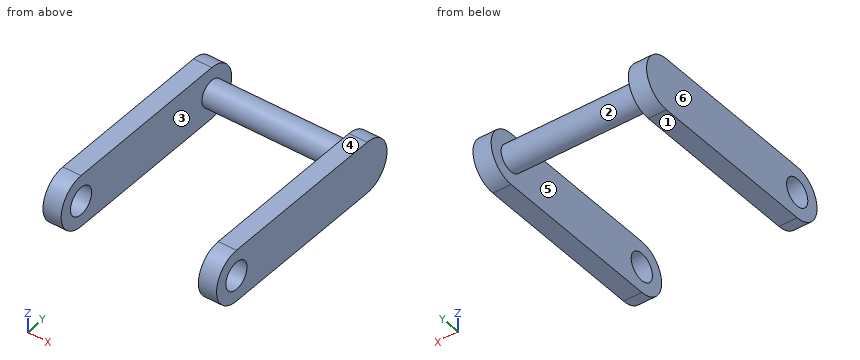
```python
from build123d import *

# Parameters (mm, degrees)
PAD139_DEPTH            = 2
SKETCH244_R             = 1.5
PAD140_DEPTH            = 16
PAD141_DEPTH            = 2
SKETCH246_R             = 1.5
PAD142_DEPTH            = 0.5
SKETCH247_R             = 1.5
PAD143_DEPTH            = 0.5
PAD143_FACE5_R          = 1.5
PAD212_DEPTH            = 0.1
PAD212_FACE4_R          = 1.5
PAD213_DEPTH            = 0.1
SKETCH353_R             = 1.6
POCKET170_DEPTH         = 22
BODY020_ROLL_ANGLE      = 90
BODY020_PLACEMENT_ANGLE = 90


with BuildPart() as part:
    # Sketch243 → Pad139 (new body)
    with BuildSketch(Plane.XY):
        with BuildLine():
            ThreePointArc((0, 3), (-3, 0), (0, -3))
            Line((0, -3), (19.75, -3))
            ThreePointArc((19.75, -3), (22.75, 0), (19.75, 3))
            Line((0, 3), (19.75, 3))
        make_face()
    extrude(amount=PAD139_DEPTH)

    # Sketch244 (on Face6 of Pad139) → Pad140 (join)
    with BuildSketch(Plane.XY.offset(2)):
        Circle(SKETCH244_R)
        with Locations((19.75, 0)):
            Circle(SKETCH244_R)
    extrude(amount=PAD140_DEPTH)

    # Sketch245 (on Face9 of Pad140) → Pad141 (join)
    with BuildSketch(Plane.XY.offset(18)):
        with BuildLine():
            ThreePointArc((0, 3), (-3, 0), (0, -3))
            Line((0, -3), (19.75, -3))
            ThreePointArc((19.75, -3), (22.75, 0), (19.75, 3))
            Line((0, 3), (19.75, 3))
        make_face()
    extrude(amount=PAD141_DEPTH)

    # Sketch246 (on Face14 of Pad141) → Pad142 (join)
    with BuildSketch(Plane.XY.offset(20)):
        Circle(SKETCH246_R)
    extrude(amount=PAD142_DEPTH)

    # Sketch247 (on Face4 of Pad142) → Pad143 (join)
    with BuildSketch(Plane(origin=(0, 0, 0), x_dir=(1, 0, 0), z_dir=(0, 0, -1))):
        Circle(SKETCH247_R)
    extrude(amount=PAD143_DEPTH)

    # Pad143 Face5 → Pad212 (add)
    with BuildSketch(Plane(origin=(9.875, 0, 2), x_dir=(0, 1, 0), z_dir=(0, 0, 1))):
        with BuildLine():
            ThreePointArc((3, 9.875), (0, 12.875), (-3, 9.875))
            Line((-3, 9.875), (-3, -9.875))
            ThreePointArc((-3, -9.875), (0, -12.875), (3, -9.875))
            Line((3, -9.875), (3, 9.875))
        make_face()
        with Locations((0, 9.875)):
            Circle(PAD143_FACE5_R, mode=Mode.SUBTRACT)
        with Locations((0, -9.875)):
            Circle(PAD143_FACE5_R, mode=Mode.SUBTRACT)
    extrude(amount=PAD212_DEPTH)

    # Pad212 Face4 → Pad213 (add)
    with BuildSketch(Plane(origin=(9.875, 0, 18), x_dir=(0, -1, 0), z_dir=(0, 0, -1))):
        with BuildLine():
            ThreePointArc((3, 9.875), (0, 12.875), (-3, 9.875))
            Line((-3, 9.875), (-3, -9.875))
            ThreePointArc((-3, -9.875), (0, -12.875), (3, -9.875))
            Line((3, -9.875), (3, 9.875))
        make_face()
        with Locations((0, 9.875)):
            Circle(PAD212_FACE4_R, mode=Mode.SUBTRACT)
        with Locations((0, -9.875)):
            Circle(PAD212_FACE4_R, mode=Mode.SUBTRACT)
    extrude(amount=PAD213_DEPTH)

    # Sketch353 (on Face3 of Pad213) → Pocket170 (cut)
    with BuildSketch(Plane.XY.offset(20.5)):
        Circle(SKETCH353_R)
    extrude(amount=-POCKET170_DEPTH, mode=Mode.SUBTRACT)


with BuildPart() as part_1:
    # Body020 roll: moved
    add(part.part.rotate(Axis((0, 0, 0), (1, 0, 0)), BODY020_ROLL_ANGLE))


with BuildPart() as part_2:
    # Body020 placement: moved
    add(part_1.part.moved(Location((28.2, -60.15, 0))).rotate(Axis((28.2, -60.15, 0), (0, 0, 1)), BODY020_PLACEMENT_ANGLE))


solid = part_2.part
```
The listing builds one solid part. Answer for the finished solid, in the listing's coordinates (mm). Face numbers are marked on the shaded views. A direction names the side the tool comes from. Give positions to 0.01 mm unless a question says otherwise; leave off trailing zeros. Loops run counter-clockwise (first coordinate to the right, second up) from the corner with the lowest first, then second, coordinate; pieces in that order, holes last. Notation, with made-up numbers: M -10.5,-8.5 L -4.5,-8.5 A20 cw -4.5,6.5 Z; hole C 43,1.25 d5. An arc over 180 degrees is marked long. One line per item, written item: value.
Q1. Flat-ended cylindrical pins translate along their axes: P1, Ø2, axis at x = 45, z = 1, coming from the +Y side; P2, Ø1.5, axis at x = 45, y = -56.5, coming from the -Z side. Find the tip coordinate at first contact, or state that the pin passes through.
Working result:
P1: stops at y = -38.9
P2: passes through
Q2. A cutting plane is placed at C-C on z = 2. Determine the outline of the cut face in (x, y), then the cut area to 3 significant figures.
Working result:
outline: M 28.2,-62.39 L 30.3,-62.39 L 30.3,-38.16 L 28.2,-38.16 Z; M 46.1,-62.39 L 48.2,-62.39 L 48.2,-38.16 L 46.1,-38.16 Z
area: 102 mm^2
Q3. For the marked faces 1 and 2, determine the directions among +Z, -Z, +X, -X, +Y, -Y from which every point of the face is accessible in a straight line to the end or side of a thin tool.
Working result:
face 1: -Z, +X, -X, +Y, -Y
face 2: none
Q4. A cutting plane is placed at A-A on z = 0. Determine the outline of the cut face in (x, y).
Working result:
outline: M 28.2,-63.15 L 30.3,-63.15 L 30.3,-61.75 L 28.2,-61.75 Z; M 28.2,-58.55 L 30.3,-58.55 L 30.3,-41.9 L 46.1,-41.9 L 46.1,-58.55 L 48.2,-58.55 L 48.2,-37.4 L 46.1,-37.4 L 46.1,-38.9 L 30.3,-38.9 L 30.3,-37.4 L 28.2,-37.4 Z; M 46.1,-63.15 L 48.2,-63.15 L 48.2,-61.75 L 46.1,-61.75 Z
Q5. A cutting plane is placed at B-B on y = -43.75. Determine the outline of the cut face in (x, z), then the cut area to 3 significant figures.
Working result:
outline: M 28.2,-3 L 30.3,-3 L 30.3,3 L 28.2,3 Z; M 46.1,-3 L 48.2,-3 L 48.2,3 L 46.1,3 Z
area: 25.2 mm^2
Q6. Determine the mould class of the marked faces 3, 4, 5 and 6 for opening direction X: +X half, -X half, draft (parallel to the pull), parting line (faces both ways), or undercut.
Working result:
face 3: undercut
face 4: draft
face 5: undercut
face 6: -X half
Q7. A cutting plane is placed at D-D on x = 44.5. Determine the outline of the cut face in (y, z).
Working result:
outline: C -40.4,0 d3
Q8. Find the intervals of material crossed by line 1 (X direction, y = -56, z = -2.5); line 2 (Z direction, x = 47, y = -60.15); line 3 (Y direction, x = 29.25, z = 0.5), in increasing order. Write a range as from..to.
Working result:
line 1: x = 28.2..30.3, 46.1..48.2
line 2: z = -3..-1.6, 1.6..3
line 3: y = -63.11..-61.67, -58.63..-37.44
